Design review of the part built by this model. Coordinates are the model's own, in mm. Face numbers are marked on the shaded views. A direction names the side the tool comes from. Give positions to 0.01 mm unless a question says otherwise; leave off trailing zeros. Loops run counter-clockwise (first coordinate to the right, second up) from the corner with the lowest first, then second, coordinate; pieces in that order, holes last. Notation, with made-up numbers: M 1.5,13.25 L 57.5,13.25 A25 ccw 57.5,27.25 Z; hole C -0.5,52 d5. An arc over 180 degrees is marked long. Use CSV: the item, a comma, the result in double quotes.
from build123d import *

# Parameters (mm, degrees)
ESBO_O2_R             = 1.5
CORTE_EXTRUS_O1_DEPTH = 10
ESBO_O3_R             = 3
CORTE_EXTRUS_O2_DEPTH = 3


with BuildPart() as part:
    # Esboço1 → Revolução2 (revolve)
    with BuildSketch(Plane.XY, mode=Mode.PRIVATE) as revolu_o2_sk:
        Polygon((0, 7), (-2.5, 7), (-2.5, 10), (15, 10), (15, 0), (0, 0), align=None)
    revolve(revolu_o2_sk.sketch.rotate(Axis((15, 0, 0), (0, 1, 0)), 180), axis=Axis((15, 0, 0), (0, 1, 0)))

    # Esboço2 → Corte-extrusão1 (cut)
    with BuildSketch(Plane(origin=(0, 0, 0), x_dir=(-1, 0, 0), z_dir=(0, -1, 0))):
        with Locations(Location((-23.5, 0, 0), (0, 0, 180))):
            Circle(ESBO_O2_R)
        with Locations(Location((-6.5, 0, 0), (0, 0, 180))):
            Circle(ESBO_O2_R)
        with BuildLine():
            Line((-16.39, 1.574134683), (-13.61, 1.574134683))
            ThreePointArc((-13.61, 1.574134683), (-15, -2.1), (-16.39, 1.574134683))
        make_face()
    extrude(amount=-CORTE_EXTRUS_O1_DEPTH, mode=Mode.SUBTRACT)

    # Esboço3 → Corte-extrusão2 (cut)
    with BuildSketch(Plane(origin=(0, 10, 0), x_dir=(1, 0, 0), z_dir=(0, 1, 0))):
        with Locations(Location((6.5, 0, 0), (0, 0, 180))):
            Circle(ESBO_O3_R)
        with Locations(Location((23.5, 0, 0), (0, 0, 180))):
            Circle(ESBO_O3_R)
    extrude(amount=-CORTE_EXTRUS_O2_DEPTH, mode=Mode.SUBTRACT)


solid = part.part
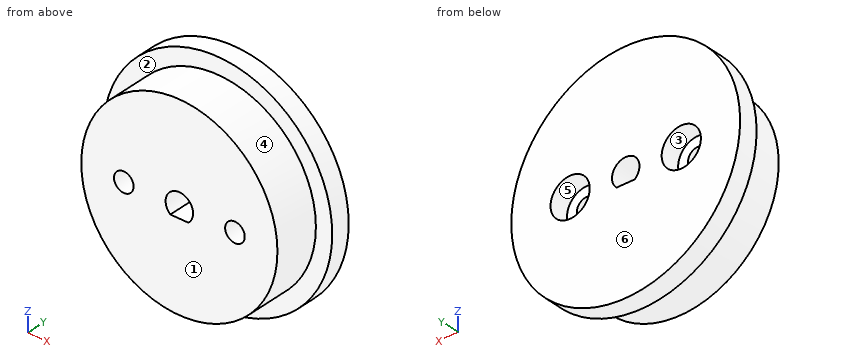
(1) We need section A-A on x = 15. State the section outline as (y, z) points, then the cut area to 3 significant figures.
A:
outline,"M 0,-15 L 7,-15 L 7,-17.5 L 10,-17.5 L 10,-1.57 L 0,-1.57 Z; M 0,2.1 L 10,2.1 L 10,17.5 L 7,17.5 L 7,15 L 0,15 Z"
area,"278 mm²"
(2) We need section C-C on y = 2. State the section outline as (x, z) points, then the cut area to 3 significant figures.
A:
outline,"C 15,0 d30; hole C 6.5,0 d3; hole M 13.61,-1.57 L 16.39,-1.57 A2.1 ccw long Z; hole C 23.5,0 d3"
area,"680 mm²"
(3) The part is to be moulded in two halves that separate along X. For the marked faces 4, 5 and 6, say which applies: released by +X, released by -X, zero draft, split by the parting line, or undercut.
A:
face 4,"split by the parting line"
face 5,"undercut"
face 6,"zero draft"
(4) Clearance check with flat-ended pins moving along their axes: P1, Ø5, axis at x = 23.5, z = 0, coming from the +Y side; P2, Ø2, axis at x = 13.5, y = 5, coming from the +Z side; P3, Ø4, axis at y = 6, z = 3, coming from the +X side. State where each tip first meets the part, or that it passes through.
A:
P1,"y = 7"
P2,"z = 14.99"
P3,"x = 32.45"
(5) We need section D-D on x = 2.5. State the section outline as (y, z) points, then the cut area to 3 significant figures.
A:
outline,"M 0,-8.29 L 7,-8.29 L 7,-12.25 L 10,-12.25 L 10,12.25 L 7,12.25 L 7,8.29 L 0,8.29 Z"
area,"190 mm²"
(6) We need section B-B on z = 0. State the section outline as (x, y) points.
A:
outline,"M -2.5,7 L 0,7 L 0,0 L 5,0 L 5,7 L 3.5,7 L 3.5,10 L -2.5,10 Z; M 8,0 L 12.9,0 L 12.9,10 L 9.5,10 L 9.5,7 L 8,7 Z; M 17.1,0 L 22,0 L 22,7 L 20.5,7 L 20.5,10 L 17.1,10 Z; M 25,0 L 30,0 L 30,7 L 32.5,7 L 32.5,10 L 26.5,10 L 26.5,7 L 25,7 Z"
(7) Wall thickness on line 1 along Y through (x, z) = (3.5, 12.5); line 2 along Z through (x, y) = (6.5, 8.9); line 3 along Y through (x, z) = (23, 2.5): over which ranges is each line inside the solid? List them lowest first. Write a range as [from, to].
A:
line 1,"[7, 10]"
line 2,"[-15.3, -3], [3, 15.3]"
line 3,"[0, 7]"
(8) Machinability: for the marked faces 1, 2 and 3, which of the approach directions +Z, -Z, +X, -X, +Y, -Y give a long, thin tool a straight path to every point of the face, cutting with its end or side? Answer none if there is none.
A:
face 1,"+Z, -Z, +X, -X, -Y"
face 2,"-Y"
face 3,"+Y"
